Read the model definition and answer for the solid it produces. Units are mm, in the model's axes. A direction names the side the tool comes from. Coordinates: 2 decimals unless noted, no trailing zeros. Write each loop counter-clockwise with the first axis right and the second up, starting at its lowest first coordinate (ties: lowest second). Pieces come first, ordered by that corner, then holes. Notation, with made-up numbers: (-23.75, -20.75) -> (-15.75, -20.75) arc R8 cw to (-15.75, -7.75) -> close; hole circle Ø3 at (7, 18). An arc over 180 degrees is marked (long way). Write item = value, one per line. Start each with the question number.
1) Section D-D (z = 15.25) is taken. Determine the outline of the cut face in (x, y), plus the area to 3 significant figures.
2) A flat-ended cylindrical pin translates along its axis: pin 1 Ø6.5 at (x, y) = (-17.75, -29.25) entering from -Z. Find the tip coordinate at first contact, or state that the pin passes through.
3) Section B-B (z = 7.25) is taken. Determine the outline of the cut face in (x, y), plus the area to 3 significant figures.
4) Section A-A (x = -2.5) is taken. Determine the outline of the cut face in (y, z) (3 decimals), plus the area to 3 significant figures.
5) Find the intervals of material crossed by line 1 along X through (y, z) = (29.25, 7); line 2 along Y through (x, z) = (-17.75, 16.25); line 3 along Y through (x, z) = (12, 16.75), in increasing order. Write a range as from..to.
6) For a pull along X with two mould halves and no side action, classify faces 3 (the face through (0, 33, 10)), 4 (the face through (-21.25, 0, 17)), 5 (the face through (14, -20, 15)) as released by +X, released by -X, zero draft, split by the parting line, or undercut.
7) Section C-C (y = 15) is taken. Determine the outline of the cut face in (x, z).
8) A tool of negligible diameter and unlimited length cuts with its end or side. For faces 1 (the face through (0, 2.5, 17)), 2 (the face through (21.25, 0, 17)), from which of +Z, -Z, +X, -X, +Y, -Y can it reach the whole face along a straight path? Write none if from no direction.
from build123d import *

# Parameters (mm, degrees)
SKETCH1_W               = 42.5
SKETCH1_H               = 66
SKETCH1_W_2             = 28
SKETCH1_H_2             = 28
BOSS_EXTRUDE1_DEPTH     = 20
CUT_EXTRUDE1_DEPTH      = 26
CUT_EXTRUDE1_DEPTH_BACK = 27
SKETCH3_R               = 44.45
SKETCH4_R               = 2
CUT_EXTRUDE2_DEPTH      = 27


with BuildPart() as part:
    # Sketch1 → Boss-Extrude1 (new body)
    with BuildSketch(Plane.XY):
        Rectangle(SKETCH1_W, SKETCH1_H)
        with Locations((0, 16.5)):
            Rectangle(SKETCH1_W_2, SKETCH1_H_2, mode=Mode.SUBTRACT)
        with Locations((0, -16.5)):
            Rectangle(SKETCH1_W_2, SKETCH1_H_2, mode=Mode.SUBTRACT)
    extrude(amount=BOSS_EXTRUDE1_DEPTH)

    # Sketch3 → Cut-Extrude1 (cut, two sides: drawn at the far end of the back side and taken through both)
    with BuildSketch(Plane(origin=(0, 0, 0), x_dir=(0, 0, -1), z_dir=(1, 0, 0)).offset(-CUT_EXTRUDE1_DEPTH_BACK)):
        with Locations((30, 0)):
            Circle(SKETCH3_R)
    extrude(amount=CUT_EXTRUDE1_DEPTH + CUT_EXTRUDE1_DEPTH_BACK, mode=Mode.SUBTRACT)

    # Sketch4 → Cut-Extrude2 (cut)
    with BuildSketch(Plane.XY.offset(20)):
        with Locations((-17.75, 29.25)):
            Circle(SKETCH4_R)
        with Locations((17.75, 29.25)):
            Circle(SKETCH4_R)
        with Locations((-17.75, -29.25)):
            Circle(SKETCH4_R)
        with Locations((17.75, -29.25)):
            Circle(SKETCH4_R)
    extrude(amount=-CUT_EXTRUDE2_DEPTH, mode=Mode.SUBTRACT)


solid = part.part
Answer key:
q1.outline = (-21.25, -33) -> (21.25, -33) -> (21.25, 33) -> (-21.25, 33) -> close; hole circle Ø4 at (-17.75, -29.25); hole circle Ø4 at (-17.75, 29.25); hole (-14, -30.5) -> (14, -30.5) -> (14, -2.5) -> (-14, -2.5) -> close; hole (-14, 2.5) -> (14, 2.5) -> (14, 30.5) -> (-14, 30.5) -> close; hole circle Ø4 at (17.75, -29.25); hole circle Ø4 at (17.75, 29.25)
q1.area = 1,190 mm^2
q2.pin_1 = 0.32
q3.outline = (-21.25, -33) -> (21.25, -33) -> (21.25, -24.25) -> (14, -24.25) -> (14, -30.5) -> (-14, -30.5) -> (-14, -24.25) -> (-21.25, -24.25) -> close; (-21.25, 24.25) -> (-14, 24.25) -> (-14, 30.5) -> (14, 30.5) -> (14, 24.25) -> (21.25, 24.25) -> (21.25, 33) -> (-21.25, 33) -> close; hole circle Ø4 at (-17.75, -29.25); hole circle Ø4 at (-17.75, 29.25); hole circle Ø4 at (17.75, -29.25); hole circle Ø4 at (17.75, 29.25)
q3.area = 343 mm^2
q4.outline = (-33, 0) -> (-32.799, 0) arc R44.45 cw to (-30.5, 2.335) -> (-30.5, 20) -> (-33, 20) -> close; (-2.5, 14.38) arc R44.45 cw to (2.5, 14.38) -> (2.5, 20) -> (-2.5, 20) -> close; (30.5, 2.335) arc R44.45 cw to (32.799, 0) -> (33, 0) -> (33, 20) -> (30.5, 20) -> close
q4.area = 122 mm^2
q5.line_1 = -21.25..-19.75, -15.75..-14, 14..15.75, 19.75..21.25
q5.line_2 = -33..-31.25, -27.25..27.25, 31.25..33
q5.line_3 = -33..-30.5, -2.5..2.5, 30.5..33
q6.face_3 = zero draft
q6.face_4 = released by -X
q6.face_5 = undercut
q7.outline = (-21.25, 11.84) -> (-14, 11.84) -> (-14, 20) -> (-21.25, 20) -> close; (14, 11.84) -> (21.25, 11.84) -> (21.25, 20) -> (14, 20) -> close
q8.face_1 = +Z, -Z
q8.face_2 = +Z, -Z, +X, +Y, -Y
